from build123d import *

# Parameters (mm, degrees)
F0_W     = 2.54
F0_H     = 101.6
F0_H_2   = 76.2
F0_H_3   = 38.1
F0_W_2   = 304.8
F0_H_4   = 2.54
F0_H_5   = 152.4
F0_W_3   = 152.4
F1_DEPTH = 2.54


with BuildPart() as f1:
    # F0 (on Top) → F1 (new body)
    with BuildSketch(Plane.XY):
        Polygon((203.2, -1.27), (203.2, 1.27), (200.66, 1.27), (138.43, 1.27), (135.89, 1.27), (73.66, 1.27), (71.12, 1.27), (8.89, 1.27), (6.35, 1.27), (-55.88, 1.27), (-58.42, 1.27), (-120.65, 1.27), (-123.19, 1.27), (-185.42, 1.27), (-187.96, 1.27), (-203.2, 1.27), (-203.2, -1.27), (-187.96, -1.27), (-185.42, -1.27), (-170.942, -1.27), (-168.402, -1.27), (-123.19, -1.27), (-120.65, -1.27), (-106.172, -1.27), (-103.632, -1.27), (-58.42, -1.27), (-55.88, -1.27), (-41.402, -1.27), (-38.862, -1.27), (6.35, -1.27), (8.89, -1.27), (23.368, -1.27), (25.908, -1.27), (71.12, -1.27), (73.66, -1.27), (88.138, -1.27), (90.678, -1.27), (135.89, -1.27), (138.43, -1.27), (152.908, -1.27), (155.448, -1.27), (200.66, -1.27), align=None)
        Polygon((220.218, 1.27), (203.2, 1.27), (203.2, -1.27), (217.678, -1.27), (220.218, -1.27), align=None)
        with Locations((201.93, 52.07)):
            Rectangle(F0_W, F0_H)
        with Locations((201.93, -39.37)):
            Rectangle(F0_W, F0_H_2)
        with Locations((137.16, 52.07)):
            Rectangle(F0_W, F0_H)
        with Locations((218.948, -20.32)):
            Rectangle(F0_W, F0_H_3)
        with Locations((154.178, -20.32)):
            Rectangle(F0_W, F0_H_3)
        with Locations((72.39, 52.07)):
            Rectangle(F0_W, F0_H)
        with Locations((137.16, -39.37)):
            Rectangle(F0_W, F0_H_2)
        with Locations((7.62, 52.07)):
            Rectangle(F0_W, F0_H)
        with Locations((89.408, -20.32)):
            Rectangle(F0_W, F0_H_3)
        with Locations((-57.15, 52.07)):
            Rectangle(F0_W, F0_H)
        with Locations((72.39, -39.37)):
            Rectangle(F0_W, F0_H_2)
        with Locations((-121.92, 52.07)):
            Rectangle(F0_W, F0_H)
        with Locations((24.638, -20.32)):
            Rectangle(F0_W, F0_H_3)
        with Locations((-186.69, 52.07)):
            Rectangle(F0_W, F0_H)
        with Locations((7.62, -39.37)):
            Rectangle(F0_W, F0_H_2)
        with Locations((-355.6, 0)):
            Rectangle(F0_W_2, F0_H_4)
        Polygon((-508, -1.27), (-508, 1.27), (-510.54, 1.27), (-914.4, 1.27), (-914.4, -1.27), (-911.86, -1.27), (-876.3, -1.27), (-873.76, -1.27), (-838.2, -1.27), (-835.66, -1.27), (-800.1, -1.27), (-797.56, -1.27), (-762, -1.27), (-759.46, -1.27), (-723.9, -1.27), (-721.36, -1.27), (-685.8, -1.27), (-683.26, -1.27), (-647.7, -1.27), (-645.16, -1.27), align=None)
        Polygon((-510.54, 1.27), (-508, 1.27), (-508, 382.27), (-510.54, 382.27), (-510.54, 379.73), (-510.54, 363.22), (-510.54, 360.68), (-510.54, 344.17), (-510.54, 341.63), (-510.54, 325.12), (-510.54, 322.58), (-510.54, 306.07), (-510.54, 303.53), (-510.54, 242.57), (-510.54, 240.03), (-510.54, 210.82), (-510.54, 208.28), (-510.54, 179.07), (-510.54, 176.53), (-510.54, 147.32), (-510.54, 144.78), align=None)
        with Locations((-40.132, -20.32)):
            Rectangle(F0_W, F0_H_3)
        with Locations((-646.43, -77.47)):
            Rectangle(F0_W, F0_H_5)
        with Locations((-586.74, 146.05)):
            Rectangle(F0_W_3, F0_H_4)
        with Locations((-586.74, 381)):
            Rectangle(F0_W_3, F0_H_4)
        with Locations((-57.15, -39.37)):
            Rectangle(F0_W, F0_H_2)
        with Locations((-169.672, -20.32)):
            Rectangle(F0_W, F0_H_3)
        with Locations((-913.13, -77.47)):
            Rectangle(F0_W, F0_H_5)
        with Locations((-684.53, -77.47)):
            Rectangle(F0_W, F0_H_5)
        with Locations((-586.74, 177.8)):
            Rectangle(F0_W_3, F0_H_4)
        with Locations((-586.74, 361.95)):
            Rectangle(F0_W_3, F0_H_4)
        with Locations((-104.902, -20.32)):
            Rectangle(F0_W, F0_H_3)
        with Locations((-121.92, -39.37)):
            Rectangle(F0_W, F0_H_2)
        with Locations((-875.03, -77.47)):
            Rectangle(F0_W, F0_H_5)
        with Locations((-722.63, -77.47)):
            Rectangle(F0_W, F0_H_5)
        with Locations((-586.74, 209.55)):
            Rectangle(F0_W_3, F0_H_4)
        with Locations((-586.74, 342.9)):
            Rectangle(F0_W_3, F0_H_4)
        with Locations((-836.93, -77.47)):
            Rectangle(F0_W, F0_H_5)
        with Locations((-760.73, -77.47)):
            Rectangle(F0_W, F0_H_5)
        with Locations((-586.74, 241.3)):
            Rectangle(F0_W_3, F0_H_4)
        with Locations((-586.74, 323.85)):
            Rectangle(F0_W_3, F0_H_4)
        with Locations((-798.83, -77.47)):
            Rectangle(F0_W, F0_H_5)
        with Locations((-586.74, 304.8)):
            Rectangle(F0_W_3, F0_H_4)
    extrude(amount=F1_DEPTH)


solid = f1.part
Could you check a few things on this model? Use its own coordinates, in mm. Give positions to 0.01 mm unless a question says otherwise; leave off trailing zeros. Order: outer loops, then holes, each group sorted by start corner. A loop starts at its lowest first (then second) coordinate and runs counter-clockwise, first axis right, second up.
1. Suppose I cut it at D-D (x = -210.5). List the corners of the cut face in (y, z) for me.
2. Suppose I cut it at C-C (y = 283). List the corners of the cut face in (x, z) for me, plus the area to 3 significant figures.
3. Will these pins go through, and if not, where does the flat tip stop? P1, Ø0.8, axis at x = 211.5, z = 1.5, coming from the -Y side; P2, Ø0.8, axis at x = -57, z = 1.5, coming from the +Y side.
4. Suppose I cut it at A-A (y = -111). Give the number of separate pieces and of enclosed holes in the cut face, plus the area to 3 significant figures.
5. I need wall thicknesses on L1, parallel to X at y = 250, z = 2.35; L2, parallel to Y at x = -164, z = 0.3. Which ranges of each line are inside material? Lowest first, please.
Solved:
1. outline: (-1.27, 0) - (1.27, 0) - (1.27, 2.54) - (-1.27, 2.54) - close
2. outline: (-510.54, 0) - (-508, 0) - (-508, 2.54) - (-510.54, 2.54) - close
2. area: 6.45 mm2
3. P1: stops at y = -1.27
3. P2: stops at y = 102.87
4. separate pieces: 8
4. enclosed holes: 0
4. area: 51.6 mm2
5. L1: x = -510.54 to -508
5. L2: y = -1.27 to 1.27
